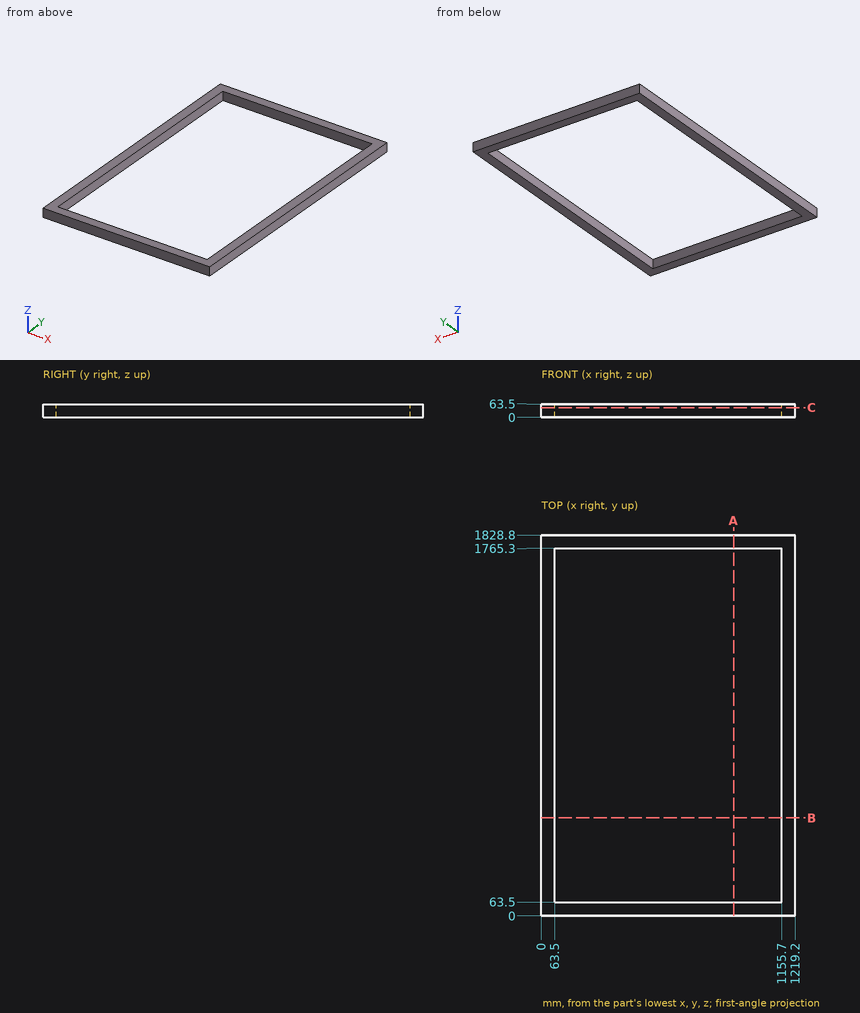
Verification items for this drawing (mm, ordinates from the low corner). Give positions to 0.01 mm unless a question says otherwise; leave off trailing zeros. Loops run counter-clockwise (first coordinate to the right, second up) from the corner with the lowest first, then second, coordinate; pieces in that order, holes last. Notation, with made-up numbers: M -39,14 L -2,14 A9 cw -2,18 Z; hole C 73,21 d3. An arc over 180 degrees is marked long. Write item = value, one per line.
(1) Sectioned sample at C-C, the plane z = 45.5. Record the cut outline in (x, y).
Answer below:
outline = M 0,0 L 1219.2,0 L 1219.2,1828.8 L 0,1828.8 Z; hole M 63.5,63.5 L 1155.7,63.5 L 1155.7,1765.3 L 63.5,1765.3 Z
(2) Sectioned sample at B-B, the plane y = 469.5. Record the cut outline in (x, z).
Answer below:
outline = M 0,0 L 63.5,0 L 63.5,63.5 L 0,63.5 Z; M 1155.7,0 L 1219.2,0 L 1219.2,63.5 L 1155.7,63.5 Z
(3) Sectioned sample at A-A, the plane x = 924.5. Record the cut outline in (y, z), plus the area to 3 significant figures.
Answer below:
outline = M 0,0 L 63.5,0 L 63.5,63.5 L 0,63.5 Z; M 1765.3,0 L 1828.8,0 L 1828.8,63.5 L 1765.3,63.5 Z
area = 8,060 mm2
(4) Material ranges on line 1 (Y direction, x = 821, z = 54); line 2 (X direction, y = 500.5, z = 53.5), recorded low to high. Write a range as [from, to].
Answer below:
line_1 = [0, 63.5], [1765.3, 1828.8]
line_2 = [0, 63.5], [1155.7, 1219.2]
